The model under review builds one solid part; all positions refer to its coordinate system, in mm. A direction names the side the tool comes from. Coordinates: 2 decimals unless noted, no trailing zeros. Write each loop counter-clockwise with the first axis right and the second up, starting at its lowest first coordinate (ties: lowest second). Pieces come first, ordered by that corner, then holes. Notation, with made-up numbers: M -33,67 L 11,67 A23 ccw 11,99 Z; hole C -24.5,35 d1. An arc over 180 degrees is marked long. Answer as a JSON object with one key per item and string values.
```python
from build123d import *

# Parameters (mm, degrees)
SKETCH1_R           = 20
BOSS_EXTRUDE1_DEPTH = 4
SKETCH2_R           = 20
SKETCH2_R_2         = 17.5
BOSS_EXTRUDE2_DEPTH = 4
SKETCH3_R           = 20
CUT_EXTRUDE1_DEPTH  = 2
SKETCH4_R           = 20
CUT_EXTRUDE2_DEPTH  = 1
SKETCH5_R           = 25
BOSS_EXTRUDE3_DEPTH = 2
BOSS_EXTRUDE4_START = 4
SKETCH6_R           = 20
SKETCH6_R_2         = 17.5
BOSS_EXTRUDE4_DEPTH = 4
SKETCH7_R           = 1.5
CUT_EXTRUDE3_DEPTH  = 16
SKETCH8_W           = 7
SKETCH8_H           = 7
CUT_EXTRUDE4_DEPTH  = 2
SKETCH9_W           = 7
SKETCH9_H           = 7
CUT_EXTRUDE5_DEPTH  = 2
SKETCH10_W          = 7
SKETCH10_H          = 7
CUT_EXTRUDE6_DEPTH  = 2
SKETCH11_R          = 24.253678372
CUT_EXTRUDE7_DEPTH  = 1
SKETCH12_R          = 1.65
CUT_EXTRUDE8_DEPTH  = 10


with BuildPart() as part:
    # Sketch1 → Boss-Extrude1 (new body)
    with BuildSketch(Plane(origin=(0, 0, 0), x_dir=(1, 0, 0), z_dir=(0, 1, 0))):
        with Locations(Location((0, 0, 0), (0, 0, 270))):
            Circle(SKETCH1_R)
    extrude(amount=BOSS_EXTRUDE1_DEPTH)

    # Sketch2 → Boss-Extrude2 (add)
    with BuildSketch(Plane(origin=(0, 4, 0), x_dir=(1, 0, 0), z_dir=(0, 1, 0))):
        with Locations(Location((0, 0, 0), (0, 0, 270))):
            Circle(SKETCH2_R)
        with Locations(Location((0, 0, 0), (0, 0, 270))):
            Circle(SKETCH2_R_2, mode=Mode.SUBTRACT)
    extrude(amount=BOSS_EXTRUDE2_DEPTH)

    # Sketch3 → Cut-Extrude1 (cut)
    with BuildSketch(Plane.XZ):
        with Locations(Location((0, 0, 0), (0, 0, 270))):
            Circle(SKETCH3_R)
    extrude(amount=-CUT_EXTRUDE1_DEPTH, mode=Mode.SUBTRACT)

    # Sketch4 → Cut-Extrude2 (cut)
    with BuildSketch(Plane(origin=(0, 2, 0), x_dir=(-1, 0, 0), z_dir=(0, -1, 0))):
        with Locations(Location((0, 0, 0), (0, 0, 90))):
            Circle(SKETCH4_R)
    extrude(amount=-CUT_EXTRUDE2_DEPTH, mode=Mode.SUBTRACT)

    # Sketch5 → Boss-Extrude3 (add)
    with BuildSketch(Plane.XZ.offset(-3)):
        with Locations(Location((0, 0, 0), (0, 0, 270))):
            Circle(SKETCH5_R)
    extrude(amount=BOSS_EXTRUDE3_DEPTH)

    # Sketch6 → Boss-Extrude4 (add)
    with BuildSketch(Plane.XZ.offset(-1).offset(BOSS_EXTRUDE4_START)):
        with Locations(Location((0, 0, 0), (0, 0, 270))):
            Circle(SKETCH6_R)
        with Locations(Location((0, 0, 0), (0, 0, 90))):
            Circle(SKETCH6_R_2, mode=Mode.SUBTRACT)
    extrude(amount=-BOSS_EXTRUDE4_DEPTH)

    # Sketch7 → Cut-Extrude3 (cut)
    with BuildSketch(Plane.XZ.offset(3)):
        with Locations(Location((-20, 0, 0), (0, 0, 272.149095627))):
            Circle(SKETCH7_R)
        with Locations(Location((-14.142135624, 14.142135624, 0), (0, 0, 227.149095627))):
            Circle(SKETCH7_R)
        with Locations(Location((0, 20, 0), (0, 0, 182.149095627))):
            Circle(SKETCH7_R)
        with Locations(Location((14.142135624, 14.142135624, 0), (0, 0, 312.850904373))):
            Circle(SKETCH7_R)
        with Locations(Location((20, 0, 0), (0, 0, 267.850904373))):
            Circle(SKETCH7_R)
        with Locations(Location((14.142135624, -14.142135624, 0), (0, 0, 222.850904373))):
            Circle(SKETCH7_R)
        with Locations(Location((0, -20, 0), (0, 0, 177.850904373))):
            Circle(SKETCH7_R)
        with Locations(Location((-14.142135624, -14.142135624, 0), (0, 0, 317.149095627))):
            Circle(SKETCH7_R)
    extrude(amount=-CUT_EXTRUDE3_DEPTH, mode=Mode.SUBTRACT)

    # Sketch8 → Cut-Extrude4 (cut)
    with BuildSketch(Plane.XZ.offset(-1)):
        with Locations((0, 10)):
            Rectangle(SKETCH8_W, SKETCH8_H)
        with Locations((0, -10)):
            Rectangle(SKETCH8_W, SKETCH8_H)
    extrude(amount=-CUT_EXTRUDE4_DEPTH, mode=Mode.SUBTRACT)

    # Sketch9 → Cut-Extrude5 (cut)
    with BuildSketch(Plane.XZ.offset(-3)):
        with Locations((0, -10)):
            Rectangle(SKETCH9_W, SKETCH9_H)
    extrude(amount=-CUT_EXTRUDE5_DEPTH, mode=Mode.SUBTRACT)

    # Sketch10 → Cut-Extrude6 (cut)
    with BuildSketch(Plane.XZ.offset(-3)):
        with Locations((0, 10)):
            Rectangle(SKETCH10_W, SKETCH10_H)
    extrude(amount=-CUT_EXTRUDE6_DEPTH, mode=Mode.SUBTRACT)

    # Sketch11 → Cut-Extrude7 (cut)
    with BuildSketch(Plane(origin=(0, 8, 0), x_dir=(1, 0, 0), z_dir=(0, 1, 0))):
        Circle(SKETCH11_R)
    extrude(amount=-CUT_EXTRUDE7_DEPTH, mode=Mode.SUBTRACT)

    # Sketch12 → Cut-Extrude8 (cut, symmetric)
    with BuildSketch(Plane(origin=(0, 3, 0), x_dir=(1, 0, 0), z_dir=(0, 1, 0))):
        with Locations(Location((20, 0, 0), (0, 0, 267.635878321))):
            Circle(SKETCH12_R)
        with Locations(Location((14.142135624, -14.142135624, 0), (0, 0, 222.635878321))):
            Circle(SKETCH12_R)
        with Locations(Location((0, -20, 0), (0, 0, 177.635878321))):
            Circle(SKETCH12_R)
        with Locations(Location((-14.142135624, -14.142135624, 0), (0, 0, 317.364121679))):
            Circle(SKETCH12_R)
        with Locations(Location((-20, 0, 0), (0, 0, 272.364121679))):
            Circle(SKETCH12_R)
        with Locations(Location((-14.142135624, 14.142135624, 0), (0, 0, 227.364121679))):
            Circle(SKETCH12_R)
        with Locations(Location((0, 20, 0), (0, 0, 182.364121679))):
            Circle(SKETCH12_R)
        with Locations(Location((14.142135624, 14.142135624, 0), (0, 0, 312.635878321))):
            Circle(SKETCH12_R)
    extrude(amount=CUT_EXTRUDE8_DEPTH, both=True, mode=Mode.SUBTRACT)


solid = part.part
```
(1) Add section A-A on x = 0. Give the boundary of the cut face in (y, z).
Results list:
{"outline": "M -3,-18.35 L 7,-18.35 L 7,-17.5 L 4,-17.5 L 4,-13.5 L 1,-13.5 L 1,-17.5 L -3,-17.5 Z; M -3,17.5 L 1,17.5 L 1,13.5 L 4,13.5 L 4,17.5 L 7,17.5 L 7,18.35 L -3,18.35 Z; M 1,-25 L 3,-25 L 3,-21.65 L 1,-21.65 Z; M 1,-6.5 L 4,-6.5 L 4,6.5 L 1,6.5 Z; M 1,21.65 L 3,21.65 L 3,25 L 1,25 Z"}
(2) Wall thickness on line 1 along X through (y, z) = (5, 0); line 2 along Z through (x, y) = (14.5, 2.25); line 3 along Y through (x, z) = (-5, 16): over which ranges is each line inside the solid? List them lowest first. Write a range as from..to.
Results list:
{"line 1": "-18.35..-17.5, 17.5..18.35", "line 2": "-20.37..-15.75, -12.53..12.53, 15.75..20.37", "line 3": "1..4"}
(3) Add section B-B on z = 0. Give the boundary of the cut face in (x, y), and give its area (3 significant figures).
Results list:
{"outline": "M -25,1 L -21.65,1 L -21.65,3 L -25,3 Z; M -18.35,-3 L -17.5,-3 L -17.5,1 L 17.5,1 L 17.5,-3 L 18.35,-3 L 18.35,7 L 17.5,7 L 17.5,4 L -17.5,4 L -17.5,7 L -18.35,7 Z; M 21.65,1 L 25,1 L 25,3 L 21.65,3 Z", "area": "135 mm²"}
(4) Add section D-D on z = 8. Give the boundary of the cut face in (x, y), and give its area (3 significant figures).
Results list:
{"outline": "M -23.69,1 L -18.33,1 L -18.33,-3 L -15.56,-3 L -15.56,1 L -3.5,1 L -3.5,4 L -15.56,4 L -15.56,7 L -18.33,7 L -18.33,3 L -23.69,3 Z; M 3.5,1 L 15.56,1 L 15.56,-3 L 18.33,-3 L 18.33,1 L 23.69,1 L 23.69,3 L 18.33,3 L 18.33,7 L 15.56,7 L 15.56,4 L 3.5,4 Z", "area": "149 mm²"}
(5) For pin 1 Ø2.5 at (x, y) = (-1.5, 3) entering from +Z; pin 2 Ø21 at (x, z) = (0, 0) entering from +Y; pin 3 Ø2 at (x, z) = (19, -15) entering from +Y, all flat-tipped, find the tip position at first contact; note any pin that passes through.
Results list:
{"pin 1": "z = 25", "pin 2": "y = 4", "pin 3": "y = 3"}
(6) Add section C-C on y = -1.5. Give the boundary of the cut face in (x, z).
Results list:
{"outline": "M -19.93,-1.65 A20 ccw -15.26,-12.93 A1.65 cw -12.93,-15.26 A20 ccw -1.65,-19.93 A1.65 cw 1.65,-19.93 A20 ccw 12.93,-15.26 A1.65 cw 15.26,-12.93 A20 ccw 19.93,-1.65 A1.65 cw 19.93,1.65 A20 ccw 15.26,12.93 A1.65 cw 12.93,15.26 A20 ccw 1.65,19.93 A1.65 cw -1.65,19.93 A20 ccw -12.93,15.26 A1.65 cw -15.26,12.93 A20 ccw -19.93,1.65 A1.65 cw Z; hole C 0,0 d35"}
(7) Draft analysis for pull direction Z (two halves, no side actions). For faces 1 (the face through (-7.6, 5, -18.5)), 2 (the face through (3.5, 2, 10)), 3 (the face through (7.734, -1.028, 18.444)), state which applies: released by +Z, released by -Z, zero draft, split by the parting line, or undercut.
Results list:
{"face 1": "released by -Z", "face 2": "undercut", "face 3": "released by +Z"}
(8) For faces 4 (the face through (-7, 3, 19)), 5 (the face through (0, 2, -6.5)), 6 (the face through (18.5, -1, 7.6)), list the 3-axis set-ups (+Z, -Z, +X, -X, +Y, -Y) from which the entire face can be reached by the end or side of a thin tool; tool diameter is ignored.
Results list:
{"face 4": "+Y", "face 5": "+Y, -Y", "face 6": "+Z, +X, -Y"}
